Autodesk Inventor part; units mm, degrees
ref_plane "YZ Plane" through (0, 0, 0) normal (1, 0, 0) x (0, 1, 0)
ref_plane "XZ Plane" through (0, 0, 0) normal (0, 1, 0) x (-1, 0, 0)
ref_plane "XY Plane" through (0, 0, 0) normal (0, 0, 1) x (1, 0, 0)
sketch "Sketch1" plane through (0, 0, 0) normal (0, 1, 0) x (-1, 0, 0)
  line L0 (27.5, 12.5) -> (-27.5, 12.5)
  line L1 (-27.5, 12.5) -> (-27.5, -12.5)
  line L2 (-27.5, -12.5) -> (27.5, -12.5)
  line L3 (27.5, -12.5) -> (27.5, 12.5)
  line L4 (27.5, 12.5) -> (-27.5, -12.5) construction
  line L5 (-27.5, 12.5) -> (27.5, -12.5) construction
  line L6 (27.5, 0) -> (17.5, 0) construction
  line L7 (17.5, 12.5) -> (17.5, 8.5) construction
  line L8 (17.5, -12.5) -> (17.5, -8.5) construction
  circle A0 centre (17.5, 8.5) radius 2.75
  circle A1 centre (17.5, -8.5) radius 2.75
  line L9 (-27.5, 12.5) -> (-22.5, 12.5) construction
  line L10 (-22.5, 12.5) -> (-22.5, -12.5)
  point P0 (0, 0)
  dimension "d0" = 55
  dimension "d1" = 25
  dimension "d2" = 10
  dimension "d3" = 4
  dimension "d4" = 4
  dimension "d5" = 5.5
  dimension "d6" = 5.5
  dimension "d7" = 5
extrude "Extrusion1" add sketch "Sketch1" against normal blind 3 contours L3 L2 L10 L0
extrude "Extrusion2" add sketch "Sketch1" against normal blind 3 contours L10 L2 L1 L0
extrude "Extrusion3" add sketch "Sketch1" along normal blind 65 contours L10 L2 L1 L0
sketch "Sketch2" plane through (0, 65, 0) normal (0, 1, 0) x (1, 0, 0)
  line L0 (27.5, -12.5) -> (-27.5, -12.5) construction
  line L1 (27.5, -12.5) -> (25, -12.5) construction
  line L2 (25, -12.5) -> (25, -10) construction
  line L3 (27.5, 12.5) -> (22.5, 12.5) construction
  line L4 (25, 12.5) -> (25, 10) construction
  circle A0 centre (25, -10) radius 0.75
  circle A1 centre (25, 10) radius 0.75
  point P0 (0, 0)
  dimension "d14" = 2.5
  dimension "d15" = 2.5
  dimension "d16" = 2.5
  dimension "d17" = 1.5
  dimension "d18" = 1.5
extrude "Extrusion4" cut sketch "Sketch2" against normal blind 20
fillet "Fillet1" radius 10 1 edges at (22.5, 0, 0)
properties part number "Camera_Wiper"
The listing builds one solid part. Answer for the finished solid, in the listing's coordinates (mm). A direction names the side the tool comes from. Coordinates: 2 decimals unless noted, no trailing zeros. Order: outer loops, then holes, each group sorted by start corner. A loop starts at its lowest first (then second) coordinate and runs counter-clockwise, first axis right, second up. Notation, with made-up numbers: (-16.75, 57) -> (-4.75, 57) arc R17 cw to (-4.75, 79) -> close; hole circle Ø3 at (63.25, 76). An arc over 180 degrees is marked (long way). Answer in a Markdown table with one row per item. Add a question column.
Item 1: Determine the mould class of faces 1 (the face through (25, 65, 0)), 2 (the face through (-14.753, -1.479, 8.621)), 3 (the face through (22.5, 37, 0)), 4 (the face through (24.45, 55.14, -10.51)) for opening direction X: +X half, -X half, draft (parallel to the pull), parting line (faces both ways), or undercut.
Item 2: Find section C-C (x = 25). Write down the section's boundary in (y, z), then the cut area to 3 significant figures.
Item 3: Find section D-D (z = 4.5). Write down the section's boundary in (x, y).
Item 4: Find section A-A (x = -17.5). Write down the section's boundary in (y, z).
Item 5: Which of the six approach directions +Z, -Z, +X, -X, +Y, -Y give full straight-line access (tool end or side, diameter ignored) to faces 5 (the face through (0, -3, 0)), 6 (the face through (24.45, 55.14, 9.49)), 7 (the face through (-7, 0, 0))?
Item 6: Find the intervals of material crossed by L1, parallel to Z at x = -17.5, y = -0.65; L2, parallel to Z at x = 25, y = 52.75; L3, parallel to X at y = 58, z = -10, in increasing order. Write a range as from..to.
Item 7: Find section B-B (z = 8.5). Write down the section's boundary in (x, y).
Item 8: Each of these flat-tipped pins is pushed along its axis until it touches: P1, Ø1.5, axis at x = 16, z = -9.5, coming from the +Y side; P2, Ø2, axis at y = 35.5, z = -6.5, coming from the -X side; P3, Ø6.5, axis at x = -17.5, z = -8.5, coming from the +Y side. Where does it stop, or does it pass through?
Result set:
| question | item | result |
|---|---|---|
| 1 | face 1 | draft |
| 1 | face 2 | undercut |
| 1 | face 3 | -X half |
| 1 | face 4 | undercut |
| 2 | outline | (-3, -12.5) -> (65, -12.5) -> (65, -10.75) -> (45, -10.75) -> (45, -9.25) -> (65, -9.25) -> (65, 9.25) -> (45, 9.25) -> (45, 10.75) -> (65, 10.75) -> (65, 12.5) -> (-3, 12.5) -> close |
| 2 | area | 1,640 mm² |
| 3 | outline | (-27.5, -3) -> (27.5, -3) -> (27.5, 65) -> (22.5, 65) -> (22.5, 10) arc R10 cw to (12.5, 0) -> (-27.5, 0) -> close |
| 4 | outline | (-3, -12.5) -> (0, -12.5) -> (0, -11.25) -> (-3, -11.25) -> close; (-3, -5.75) -> (0, -5.75) -> (0, 5.75) -> (-3, 5.75) -> close; (-3, 11.25) -> (0, 11.25) -> (0, 12.5) -> (-3, 12.5) -> close |
| 5 | face 5 | +Z, -Z, +X, -X, -Y |
| 5 | face 6 | +Y |
| 5 | face 7 | +Z, -Z, -X, +Y |
| 6 | L1 | z = -12.5..-11.25, -5.75..5.75, 11.25..12.5 |
| 6 | L2 | z = -12.5..-10.75, -9.25..9.25, 10.75..12.5 |
| 6 | L3 | x = 22.5..24.25, 25.75..27.5 |
| 7 | outline | (-27.5, -3) -> (-20.25, -3) -> (-20.25, 0) -> (-27.5, 0) -> close; (-14.75, -3) -> (27.5, -3) -> (27.5, 65) -> (22.5, 65) -> (22.5, 10) arc R10 cw to (12.5, 0) -> (-14.75, 0) -> close |
| 8 | P1 | stops at y = 0.95 |
| 8 | P2 | stops at x = 22.5 |
| 8 | P3 | stops at y = 0 |
